```python
from build123d import *

# Parameters (mm, degrees)
F0_W     = 110
F0_H     = 98
F0_W_2   = 107
F0_H_2   = 95
F0_W_3   = 100
F0_H_3   = 5
F1_DEPTH = 2
F2_DEPTH = 35
F3_W     = 5
F3_H     = 30
F4_DEPTH = 150


with BuildPart() as f1:
    # F0 (on Top) → F1 (new body)
    with BuildSketch(Plane.XY):
        Rectangle(F0_W, F0_H)
        Rectangle(F0_W_2, F0_H_2, mode=Mode.SUBTRACT)
        Rectangle(F0_W_2, F0_H_2)
        with Locations((0, -39.2500515282)):
            Rectangle(F0_W_3, F0_H_3, mode=Mode.SUBTRACT)
        with Locations((0, -29.2500515282)):
            Rectangle(F0_W_3, F0_H_3, mode=Mode.SUBTRACT)
        with Locations((0, -19.2500515282)):
            Rectangle(F0_W_3, F0_H_3, mode=Mode.SUBTRACT)
        with Locations((0, -9.2500515282)):
            Rectangle(F0_W_3, F0_H_3, mode=Mode.SUBTRACT)
        with Locations((0, 0.7499484718)):
            Rectangle(F0_W_3, F0_H_3, mode=Mode.SUBTRACT)
        with Locations((0, 10.7499484718)):
            Rectangle(F0_W_3, F0_H_3, mode=Mode.SUBTRACT)
        with Locations((0, 20.7499484718)):
            Rectangle(F0_W_3, F0_H_3, mode=Mode.SUBTRACT)
        with Locations((0, 30.7499484718)):
            Rectangle(F0_W_3, F0_H_3, mode=Mode.SUBTRACT)
        with Locations((0, 40.7499484718)):
            Rectangle(F0_W_3, F0_H_3, mode=Mode.SUBTRACT)
    extrude(amount=F1_DEPTH)

    # F0 (on Top) → F2 (join)
    with BuildSketch(Plane.XY):
        Rectangle(F0_W, F0_H)
        Rectangle(F0_W_2, F0_H_2, mode=Mode.SUBTRACT)
    extrude(amount=F2_DEPTH)

    # F3 (on face) → F4 (cut)
    with BuildSketch(Plane.XZ.offset(49)):
        with Locations((-36.8548509181, 17.5)):
            Rectangle(F3_W, F3_H)
        with Locations((-47.3548509181, 17.5)):
            Rectangle(F3_W, F3_H)
        with Locations((-26.3548509181, 17.5)):
            Rectangle(F3_W, F3_H)
        with Locations((-15.8548509181, 17.5)):
            Rectangle(F3_W, F3_H)
        with Locations((-5.3548509181, 17.5)):
            Rectangle(F3_W, F3_H)
        with Locations((5.1451490819, 17.5)):
            Rectangle(F3_W, F3_H)
        with Locations((15.6451490819, 17.5)):
            Rectangle(F3_W, F3_H)
        with Locations((26.1451490819, 17.5)):
            Rectangle(F3_W, F3_H)
        with Locations((36.6451490819, 17.5)):
            Rectangle(F3_W, F3_H)
        with Locations((47.1451490819, 17.5)):
            Rectangle(F3_W, F3_H)
    extrude(amount=-F4_DEPTH, mode=Mode.SUBTRACT)


solid = f1.part
```
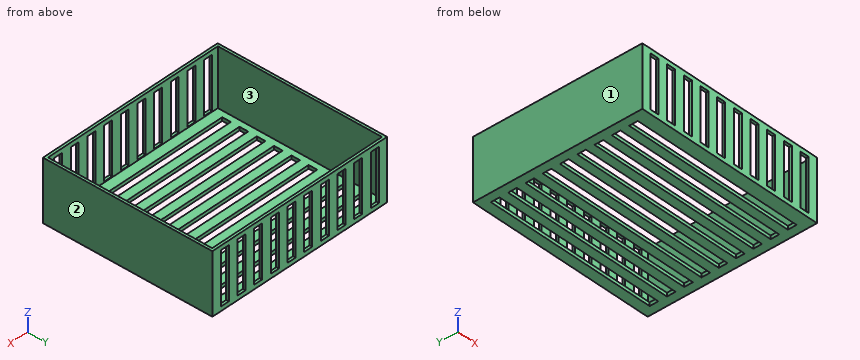
Here's how the part is built. I have some questions about the finished solid (model axes, mm). Face numbers are marked on the shaded views. Give positions to 0.01 mm unless a question says otherwise; leave off trailing zeros. Order: outer loops, then holes, each group sorted by start corner. A loop starts at its lowest first (then second) coordinate and runs counter-clockwise, first axis right, second up. Notation, with made-up numbers: (69.5, 21) -> (109.5, 21) arc R37 ccw to (109.5, 57) -> close; hole circle Ø11 at (78.5, 85.5). An arc over 180 degrees is marked (long way). Use CSV: the item, a comma, the result in double quotes. Start each with the question number.
Item 1: Suppose I cut it at A-A (y = 41). List the corners of the cut face in (x, z) for me, and give its area (3 significant figures).
Item 2: I'm going to push a flat-ended pin straight in: P1, Ø6, axis at x = -9.5, y = -4, coming from the +Z side. Where does the tip first touch, or does it pass through?
Item 3: Thinking about a two-plate mould opening in X: for the marked faces 1, 2 and 3, which applies, pulls with the +X half, pulls with the -X half, needs draft (parallel to the pull), parting line crosses it, or undercut?
Item 4: If I drill on probe 1 along Y at (x, z) = (-0.5, 21); probe 2 along X at (y, z) = (12, 21.5); probe 3 along Z at (x, y) = (-23, 16.5), over which ranges is the centre line in solid material (lowest first)? Write a range as [from, to].
Item 5: Suppose I cut it at B-B (x = -17). Give the number of separate pieces and of enclosed holes in the cut face, and give its area (3 significant figures).
Item 6: Suppose I cut it at C-C (y = -5). List the corners of the cut face in (x, z) for me, and give its area (3 significant figures).
Answer block:
1,outline,"(-55, 0) -> (-50, 0) -> (-50, 2) -> (-53.5, 2) -> (-53.5, 35) -> (-55, 35) -> close; (50, 0) -> (55, 0) -> (55, 35) -> (53.5, 35) -> (53.5, 2) -> (50, 2) -> close"
1,area,"119 mm^2"
2,P1,"stops at z = 2"
3,face 1,"pulls with the -X half"
3,face 2,"pulls with the +X half"
3,face 3,"undercut"
4,probe 1,"y = [-49, -47.5], [47.5, 49]"
4,probe 2,"x = [-55, -53.5], [53.5, 55]"
4,probe 3,"z = [0, 2]"
5,separate pieces,"12"
5,enclosed holes,"0"
5,area,"115 mm^2"
6,outline,"(-55, 0) -> (55, 0) -> (55, 35) -> (53.5, 35) -> (53.5, 2) -> (-53.5, 2) -> (-53.5, 35) -> (-55, 35) -> close"
6,area,"319 mm^2"
